Source: CAD feature listing. Evaluate the final solid. Frame: model axes, mm. A direction names the side the tool comes from. Round coordinates to 2 decimals unless told otherwise and drop trailing zeros. Loops run counter-clockwise (first coordinate to the right, second up) from the corner with the lowest first, then second, coordinate; pieces in that order, holes last. Notation, with made-up numbers: M 29.25,53 L 54.25,53 A7 cw 54.25,59 Z; hole C 56,49.5 d11. An arc over 180 degrees is marked long. Answer as a JSON object with one key per item and string values.
from build123d import *

# Parameters (mm, degrees)
BLANKSKE_W        = 17
BLANKSKE_H        = 11
BLANK_DEPTH       = 6
TOOTHCUTSIM_DEPTH = 22.118712082
TEETHCUTS_COUNT   = 6
TEETHCUTS_PITCH   = 3.14159265
SKETCH_1_W        = 6
SKETCH_1_H        = 11
EXTRUDE_1_DEPTH   = 30
SKETCH_2_W        = 16
SKETCH_2_H        = 100
EXTRUDE_2_DEPTH   = 5


with BuildPart() as part:
    # BlankSke → Blank (new body)
    with BuildSketch(Plane.XY):
        with Locations((8.5, 5.5)):
            Rectangle(BLANKSKE_W, BLANKSKE_H)
    extrude(amount=-BLANK_DEPTH)

    # TooCutSkeSim → ToothCutSim (cut, through all)
    with BuildSketch(Plane.XY):
        Polygon((0.44443537, 8.75), (-0.44443537, 8.75), (-1.272613241, 11.0254), (1.272613241, 11.0254), align=None)
    toothcutsim = extrude(amount=-TOOTHCUTSIM_DEPTH, mode=Mode.SUBTRACT)

    # TeethCuts: ToothCutSim ×6
    with Locations(*[(i * TEETHCUTS_PITCH, 0, 0) for i in range(1, TEETHCUTS_COUNT)]):
        add(toothcutsim, mode=Mode.SUBTRACT)

    # 草图1 → 凸台-拉伸1 (add)
    with BuildSketch(Plane(origin=(17, 0, 0), x_dir=(0, 0, -1), z_dir=(1, 0, 0))):
        with Locations((3, 5.5)):
            Rectangle(SKETCH_1_W, SKETCH_1_H)
    extrude(amount=EXTRUDE_1_DEPTH)

    # 草图2 → 凸台-拉伸2 (add)
    with BuildSketch(Plane(origin=(47, 0, 0), x_dir=(0, 0, -1), z_dir=(1, 0, 0))):
        with Locations((3, 5.5)):
            Rectangle(SKETCH_2_W, SKETCH_2_H)
    extrude(amount=EXTRUDE_2_DEPTH)


solid = part.part
Item 1: Section A-A on y = 5. Return the cut outline in (x, z), then the cut area to 3 significant figures.
Answer sheet:
{"outline": "M 0,-6 L 47,-6 L 47,-11 L 52,-11 L 52,5 L 47,5 L 47,0 L 0,0 Z", "area": "362 mm²"}
Item 2: Access query for faces 1 (the flat face through (23, 5, 0)), 2 (the flat face through (23, 0, -3)), 3 (the flat face through (52, 6, -3)), 4 (the flat face through (49, 5, 5)), 5 (the flat face through (10.284, 9.891, -2.958)). Directions: +Z, -Z, +X, -X, +Y, -Y. A direction counts if a zero-diameter tool reaches every point of the face in a straight line with its end or side. Return the directions, or none.
Answer sheet:
{"face 1": "+Z, -X, +Y, -Y", "face 2": "+Z, -Z, -X, -Y", "face 3": "+Z, -Z, +X, +Y, -Y", "face 4": "+Z, +X, -X, +Y, -Y", "face 5": "+Z, -Z, +Y"}
Item 3: Section C-C on x = 37.5. Return the cut outline in (y, z), then the cut area to 3 significant figures.
Answer sheet:
{"outline": "M 0,-6 L 11,-6 L 11,0 L 0,0 Z", "area": "66.0 mm²"}
Item 4: Pull-direction query (X, two-part tool) for faces 6 (the flat face through (0.86, 9.89, -2.96)), 7 (the flat face through (23, 5, -6)), 8 (the flat face through (5.435, 9.859, -2.958)), 9 (the flat face through (8.577, 9.859, -2.958)); classes: pulls with the +X half, pulls with the -X half, needs draft (parallel to the pull), parting line crosses it, or undercut.
Answer sheet:
{"face 6": "pulls with the -X half", "face 7": "needs draft", "face 8": "undercut", "face 9": "undercut"}
Item 5: Contact query for flat-ended pins moving along their axis: pin 1 Ø5 at (x, z) = (12, -3) entering from +Y; pin 2 Ø5 at (y, z) = (-4, -4.5) entering from -X; pin 3 Ø3 at (x, z) = (26.5, -3) entering from -Y. Output: stop coordinate, or through.
Answer sheet:
{"pin 1": "stops at y = 11", "pin 2": "stops at x = 47", "pin 3": "stops at y = 0"}
Item 6: Line query: probe 1 along X at (y, z) = (-25.5, 1.5); probe 2 along Y at (x, z) = (30, -4.75). Output: solid intervals per line, ascending. Write a range as from..to.
Answer sheet:
{"probe 1": "x = 47..52", "probe 2": "y = 0..11"}
Item 7: Section D-D on z = -8.5. Return the cut outline in (x, y), then the cut area to 3 significant figures.
Answer sheet:
{"outline": "M 47,-44.5 L 52,-44.5 L 52,55.5 L 47,55.5 Z", "area": "500 mm²"}
